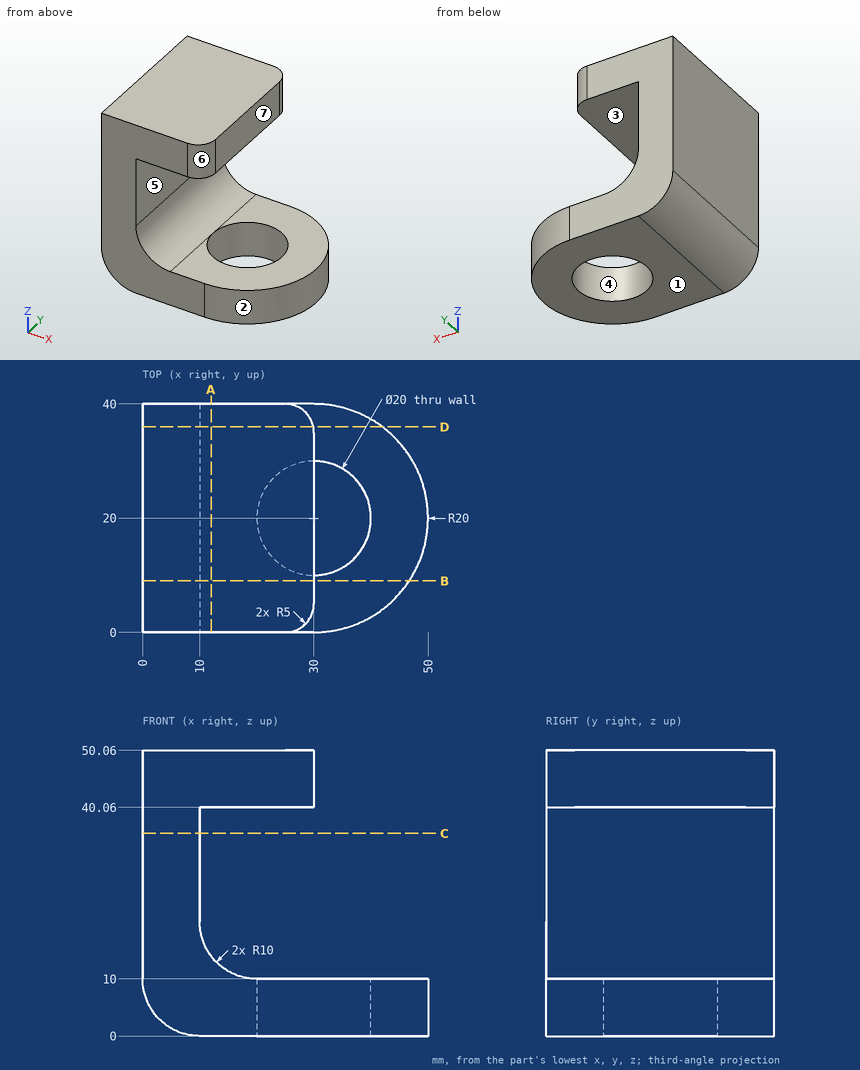
Geometry: see drawing. Coordinates: mm, zero at the bounding-box minimum. A direction names the side the tool comes from. Round coordinates to 2 decimals unless told otherwise and drop trailing zeros. Write each loop counter-clockwise with the first axis right and the second up, starting at its lowest first coordinate (ties: lowest second). Pieces come first, ordered by that corner, then holes.
1) Cut plane C-C (z = 35.5). Return the cut outline in (x, y).
2) Reachability of the marked faces 4, 5, 6 and 7 from +Z, -Z, +X, -X, +Y, -Y: full face, straight path, thin tool, end or side. Return the list, or none.
3) Draft query along Z for the marked faces 1, 2 and 3. Return one class per face: pulls with the +Z half, pulls with the -Z half, needs draft (parallel to the pull), parting line crosses it, or undercut.
4) Contact query for flat-ended pins moving along their axis: P1, Ø1, axis at y = 5.5, z = 5, coming from the +X side; P2, Ø5, axis at y = 26.5, z = 20.5, coming from the -X side; P3, Ø5, axis at y = 19.5, z = 44.5, coming from the +X side; P4, Ø6, axis at y = 32.5, z = 35.5, coming from the +X side. Output: stop coordinate, or through.
5) Cut plane B-B (y = 9). Return the cut outline in (x, z), then the cut area to 3 significant figures.
6) Cut plane A-A (x = 12). Return the cut outline in (y, z), then the cut area to 3 significant figures.
7) Ray query, L1, parallel to Y at x = 30, z = 6; L2, parallel to Z at x = 24, y = 8.5; L3, parallel to X at y = 28.5, z = 43. Return the intervals inside material, ascending.
8) Cut plane D-D (y = 36). Return the cut outline in (x, z), then the cut area to 3 significant figures.
Geometry says:
1. outline: (0, 0) - (10, 0) - (10, 40) - (0, 40) - close
2. face 4: -Z
2. face 5: +X, +Y, -Y
2. face 6: +Z, +X, -Y
2. face 7: +Z, +X, +Y, -Y
3. face 1: pulls with the -Z half
3. face 2: needs draft
3. face 3: undercut
4. P1: stops at x = 44.28
4. P2: stops at x = 0
4. P3: stops at x = 30
4. P4: stops at x = 10
5. outline: (0, 10) arc R10 ccw to (10, 0) - (46.7, 0) - (46.7, 10) - (20, 10) arc R10 cw to (10, 20) - (10, 40.06) - (30, 40.06) - (30, 50.06) - (0, 50.06) - close
5. area: 1,070 mm2
6. outline: (0, 0) - (40, 0) - (40, 14) - (0, 14) - close; (0, 40.06) - (40, 40.06) - (40, 50.06) - (0, 50.06) - close
6. area: 960 mm2
7. L1: y = 0 to 10, 30 to 40
7. L2: z = 0 to 10, 40.06 to 50.06
7. L3: x = 0 to 30
8. outline: (0, 10) arc R10 ccw to (10, 0) - (42, 0) - (42, 10) - (20, 10) arc R10 cw to (10, 20) - (10, 40.06) - (29.9, 40.06) - (29.9, 50.06) - (0, 50.06) - close
8. area: 1,020 mm2
